from build123d import *

# Parameters (mm, degrees)
BOSS_EXTRUDE2_DEPTH = 25
FILLET1_R           = 45
SKETCH7_R           = 35
SKETCH7_R_2         = 19.025
BOSS_EXTRUDE3_DEPTH = 114
SKETCH8_R           = 35
SKETCH8_R_2         = 19.025
BOSS_EXTRUDE4_DEPTH = 51
BOSS_EXTRUDE5_START = 76
BOSS_EXTRUDE5_DEPTH = 76
CUT_EXTRUDE1_START  = -38
CUT_EXTRUDE1_DEPTH  = 19
CUT_EXTRUDE2_START  = -102
CUT_EXTRUDE2_DEPTH  = 19
BOSS_EXTRUDE6_REACH = 274.283
BOSS_EXTRUDE7_REACH = 266.785
SKETCH12_R          = 9.5
CUT_EXTRUDE3_DEPTH  = 185.082182907
FILLET2_R           = 3


# Read off the part's stored shape, not the designer's step: Cut-Extrude1, Cut-Extrude2
with BuildPart() as part:
    # Sketch2 → Boss-Extrude2 (new body)
    with BuildSketch(Plane(origin=(0, 0, 0), x_dir=(1, 0, 0), z_dir=(0, 1, 0))):
        Polygon((-100, -106.5), (-100, -4.5), (62, -4.5), (62, 106.5), (100, 106.5), (100, -106.5), align=None)
    extrude(amount=BOSS_EXTRUDE2_DEPTH)

    # Fillet1
    fillet1_edges = [part.edges().sort_by_distance(p)[0] for p in [
        (62, 12.5, 4.5),
    ]]
    fillet(fillet1_edges, radius=FILLET1_R)



with BuildPart() as body_2:
    # Sketch7 → Boss-Extrude3 (new body)
    with BuildSketch(Plane.XY.offset(106.5)):
        with Locations((-17, 102)):
            Circle(SKETCH7_R)
        with Locations((-17, 102)):
            Circle(SKETCH7_R_2, mode=Mode.SUBTRACT)
    extrude(amount=-BOSS_EXTRUDE3_DEPTH)


with BuildPart() as body_3:
    # Sketch8 → Boss-Extrude4 (new body)
    with BuildSketch(Plane(origin=(100, 0, 0), x_dir=(0, 0, -1), z_dir=(1, 0, 0))):
        with Locations((71.5, 102)):
            Circle(SKETCH8_R)
        with Locations((71.5, 102)):
            Circle(SKETCH8_R_2, mode=Mode.SUBTRACT)
    extrude(amount=-BOSS_EXTRUDE4_DEPTH)


with BuildPart() as part_1:
    add(part.part)

    add(body_2.part)  # Boss-Extrude5 merges body 2

    add(body_3.part)  # Boss-Extrude5 merges body 3
    # Sketch9 → Boss-Extrude5 (add)
    with BuildSketch(Plane(origin=(0, 25, 0), x_dir=(1, 0, 0), z_dir=(0, 1, 0)).offset(BOSS_EXTRUDE5_START)):
        with BuildLine():
            Line((17, -4.5), (-52, -4.5))
            Line((-52, -4.5), (-52, -23.5))
            Line((-52, -23.5), (17, -23.5))
            ThreePointArc((17, -23.5), (62.254833996, -4.754833996), (81, 40.5))
            Line((81, 40.5), (81, 106.5))
            Line((81, 106.5), (62, 106.5))
            Line((62, 106.5), (62, 40.5))
            ThreePointArc((62, 40.5), (48.819805153, 8.680194847), (17, -4.5))
        make_face()
    extrude(amount=-BOSS_EXTRUDE5_DEPTH)

    # Cut-Extrude1 outline → Cut-Extrude1 (cut)
    with BuildSketch(Plane(origin=(100, 0, 0), x_dir=(0, 0, -1), z_dir=(1, 0, 0)).offset(CUT_EXTRUDE1_START)):
        with BuildLine():
            Line((90.498700613, 101), (52.501299387, 101))
            ThreePointArc((52.501299387, 101), (71.5, 82.975), (90.498700613, 101))
        make_face()
    extrude(amount=CUT_EXTRUDE1_DEPTH, mode=Mode.SUBTRACT)

    # Cut-Extrude2 outline → Cut-Extrude2 (cut)
    with BuildSketch(Plane.XY.offset(106.5).offset(CUT_EXTRUDE2_START)):
        with BuildLine():
            ThreePointArc((-35.998700613, 101), (-17, 82.975), (1.998700613, 101))
            Line((1.998700613, 101), (-35.998700613, 101))
        make_face()
    extrude(amount=CUT_EXTRUDE2_DEPTH, mode=Mode.SUBTRACT)

    # Sketch10 → Boss-Extrude6 (add, up to next)
    with BuildSketch(Plane.XY.offset(106.5), mode=Mode.PRIVATE) as boss_extrude6_sk1:
        with BuildLine():
            Line((-26.5, 25), (-7.5, 25))
            Line((-7.5, 25), (-7.5, 68.313949475))
            ThreePointArc((-7.5, 68.313949475), (-17, 67), (-26.5, 68.313949475))
            Line((-26.5, 68.313949475), (-26.5, 25))
        make_face()
    boss_extrude6_tool1 = extrude(boss_extrude6_sk1.sketch, amount=-BOSS_EXTRUDE6_REACH, mode=Mode.PRIVATE) - part_1.part
    add(boss_extrude6_tool1.solids().sort_by_distance((-17, 46.219119, 106.5))[0])

    # Sketch11 → Boss-Extrude7 (add, up to next)
    with BuildSketch(Plane(origin=(100, 0, 0), x_dir=(0, 0, -1), z_dir=(1, 0, 0)), mode=Mode.PRIVATE) as boss_extrude7_sk1:
        with BuildLine():
            Line((62, 25), (81, 25))
            Line((81, 25), (81, 68.313949475))
            ThreePointArc((81, 68.313949475), (71.5, 67), (62, 68.313949475))
            Line((62, 68.313949475), (62, 25))
        make_face()
    boss_extrude7_tool1 = extrude(boss_extrude7_sk1.sketch, amount=-BOSS_EXTRUDE7_REACH, mode=Mode.PRIVATE) - part_1.part
    add(boss_extrude7_tool1.solids().sort_by_distance((100, 46.219119, -71.5))[0])

    # Sketch12 → Cut-Extrude3 (cut, through all)
    with BuildSketch(Plane(origin=(0, 25, 0), x_dir=(1, 0, 0), z_dir=(0, 1, 0))):
        with Locations(Location((68, -49.5, 0), (0, 0, 270))):
            Circle(SKETCH12_R)
        with Locations(Location((68, -87.5, 0), (0, 0, 270))):
            Circle(SKETCH12_R)
        with Locations(Location((-84, -49.5, 0), (0, 0, 270))):
            Circle(SKETCH12_R)
        with Locations(Location((-84, -87.5, 0), (0, 0, 270))):
            Circle(SKETCH12_R)
    extrude(amount=-CUT_EXTRUDE3_DEPTH, mode=Mode.SUBTRACT)

    # Fillet2
    fillet2_edges = [part_1.edges().sort_by_distance(p)[0] for p in [
        (-52, 63, 4.5),
        (-7.5, 46.656974737, 23.5),
        (-7.5, 46.656974737, 106.5),
        (4.75, 25, 23.5),
        (81, 25, -51.25),
        (47.739784514, 101, -7.635647762),
        (-26.5, 25, 65),
        (-52, 25, 14),
        (-39.25, 25, 23.5),
        (-26.5, 46.656974737, 23.5),
        (-76, 25, 4.5),
        (-100, 25, 55.5),
        (-63.25, 25, 106.5),
        (81, 46.656974737, -81),
        (81, 46.656974737, -62),
        (100, 12.5, -106.5),
        (100, 25, -93.75),
        (100, 46.656974737, -81),
        (100, 46.656974737, -62),
        (61.180922368, 101, 5.803845399),
        (-26.5, 46.656974737, 106.5),
        (100, 25, 22.25),
        (46.25, 25, 106.5),
        (-7.5, 25, 65),
        (62.254833996, 25, 4.754833996),
    ]]
    fillet(fillet2_edges, radius=FILLET2_R)


solid = part_1.part
Can you work these out from the model? Positions are in its coordinate system, mm. A direction names the side the tool comes from. Coordinates: 2 decimals unless noted, no trailing zeros. Order: outer loops, then holes, each group sorted by start corner. A loop starts at its lowest first (then second) coordinate and runs counter-clockwise, first axis right, second up. Notation, with made-up numbers: (9, 42.25) - (54, 42.25) arc R19 ccw to (54, 49.25) - close; hole circle Ø4 at (55.25, 61.25). An arc over 180 degrees is marked (long way). Answer as a JSON object with one key per item and string values. Group by question number.
Q1. On a 3-axis mill with a long thin cutter (end or side, diameter ignored), from which of +Z, -Z, +X, -X, +Y, -Y can I reach the whole of each face in a straight line? I mean faces 1 (the face through (74.86, 136.7, -66.94)), 2 (the face through (49, 87, -87)), 3 (the face through (58, 25, 56)). Say none if no direction works.
Q2. Imagine slicing it at D-D (x = -17). Please give me the cut outline in (y, z) (3 decimals), and give its area (3 significant figures).
Q3. I need wall thicknesses on line 1 (X direction, y = 13.5, z = 87.5); line 2 (X direction, y = 13, z = 89); line 3 (Y direction, x = 85, z = -85.5). Which ranges of each line are inside material? Lowest first, please. Write a range as from..to.
Q4. Will these pins go through, and if not, where does the flat tip stop? P1, Ø8, axis at x = 54.5, z = 59, coming from the +Y side; P2, Ø13, axis at x = 88.5, z = -88, coming from the +Y side; P3, Ø18, axis at y = 60.5, z = -90.5, coming from the +X side.
Q5. We'd pull the mould along Y, two halves only. Please class faces 4 (the face through (-41, 57, 23.5)), 5 (the face through (-15, 49, 106.5)), 6 (the face through (24, 0, 22)): +Y half, -Y half, draft (parallel to the pull), parting line (faces both ways), or undercut.
Q6. Imagine slicing it at B-B (z = -71.5). Please give me the cut outline in (x, y) (3 decimals), and give its area (3 significant figures).
Q7. Imagine slicing it at A-A (x = -84). Please give me the cut outline in (y, z).
Q8. Imagine slicing it at C-C (y = 40). Please give me the cut outline in (x, z).
Determined:
{
 "1": {"face 1": "none", "face 2": "-Z, -X, +Y, -Y", "face 3": "+Z, +X"},
 "2": {"outline": "(0, 4.5) - (67, 4.5) - (67, -7.5) - (82.975, -7.5) - (82.975, 106.5) - (0, 106.5) - close; (121.025, -7.5) - (137, -7.5) - (137, 106.5) - (121.025, 106.5) - close", "area": "10,500 mm2"},
 "3": {"line 1": "x = -100..-93.5, -74.5..58.5, 77.5..100", "line 2": "x = -100..-93.38, -74.62..58.62, 77.38..100", "line 3": "y = 0..25, 69.92..89.12, 114.88..134.08"},
 "4": {"P1": "stops at y = 25", "P2": "stops at y = 135.54", "P3": "stops at x = 82.34"},
 "5": {"face 4": "undercut", "face 5": "draft", "face 6": "-Y half"},
 "6": {"outline": "(49, 67) - (62, 67) - (62, 0) - (100, 0) - (100, 82.975) - (49, 82.975) - close; (49, 121.025) - (100, 121.025) - (100, 137) - (49, 137) - close", "area": "4,180 mm2"},
 "7": {"outline": "(0, 4.5) - (22, 4.5) arc R3 ccw to (25, 7.5) - (25, 40) - (0, 40) - close; (0, 59) - (25, 59) - (25, 78) - (0, 78) - close; (0, 97) - (25, 97) - (25, 103.5) arc R3 ccw to (22, 106.5) - (0, 106.5) - close"},
 "8": {"outline": "(-52, 7.5) arc R3 ccw to (-49, 4.5) - (17, 4.5) arc R45 cw to (62, -40.5) - (62, -106.5) - (81, -106.5) - (81, -84) arc R3 cw to (84, -81) - (97, -81) arc R3 ccw to (100, -78) - (100, -65) arc R3 ccw to (97, -62) - (84, -62) arc R3 cw to (81, -59) - (81, -40.5) arc R64 ccw to (17, 23.5) - (-4.5, 23.5) arc R3 cw to (-7.5, 26.5) - (-7.5, 103.5) arc R3 ccw to (-10.5, 106.5) - (-23.5, 106.5) arc R3 ccw to (-26.5, 103.5) - (-26.5, 26.5) arc R3 cw to (-29.5, 23.5) - (-52, 23.5) - close"}
}
